Geometry check sheet. Reference: the model listing, model coordinates, mm. A direction names the side the tool comes from. Round coordinates to 2 decimals unless told otherwise and drop trailing zeros. Write each loop counter-clockwise with the first axis right and the second up, starting at its lowest first coordinate (ties: lowest second). Pieces come first, ordered by that corner, then holes.
from build123d import *

# Parameters (mm, degrees)
ESQUISSE1_R             = 2.25
BOSS_EXTRU_1_DEPTH      = 5
BOSS_EXTRU_2_START      = -21
BOSS_EXTRU_2_DEPTH      = 21
ESQUISSE4_W             = 13
ESQUISSE4_H             = 46
ENL_V_MAT_EXTRU_2_DEPTH = 16
ESQUISSE9_W             = 16
ESQUISSE9_H             = 36
BOSS_EXTRU_3_DEPTH      = 3
ESQUISSE10_W            = 4
ESQUISSE10_H            = 16
ENL_V_MAT_EXTRU_6_DEPTH = 43
CONG_1_R                = 2
ESQUISSE11_R            = 2.1
ENL_V_MAT_EXTRU_7_DEPTH = 43


with BuildPart() as part:
    # Esquisse1 → Boss.-Extru.1 (new body)
    with BuildSketch(Plane.XY):
        with BuildLine():
            Line((-7.4, 36), (-7.4, 0))
            Line((-7.4, 0), (7, 0))
            ThreePointArc((7, 0), (9.121320344, 0.878679656), (10, 3))
            Line((10, 3), (10, 33))
            ThreePointArc((10, 33), (9.121320344, 35.121320344), (7, 36))
            Line((7, 36), (-7.4, 36))
        make_face()
        with Locations((2, 8)):
            Circle(ESQUISSE1_R, mode=Mode.SUBTRACT)
        with Locations((2, 28)):
            Circle(ESQUISSE1_R, mode=Mode.SUBTRACT)
    extrude(amount=BOSS_EXTRU_1_DEPTH)

    # Esquisse2 → Boss.-Extru.2 (add)
    with BuildSketch(Plane.XY.offset(5).offset(BOSS_EXTRU_2_START)):
        with BuildLine():
            Line((10, 3), (10, 33))
            ThreePointArc((10, 33), (9.121320344, 35.121320344), (7, 36))
            Line((7, 36), (11, 36))
            Line((11, 36), (11, 41))
            Line((11, 41), (24, 41))
            Line((24, 41), (24, -5))
            Line((24, -5), (11, -5))
            Line((11, -5), (11, 0))
            Line((11, 0), (7, 0))
            ThreePointArc((7, 0), (9.121320344, 0.878679656), (10, 3))
        make_face()
    extrude(amount=BOSS_EXTRU_2_DEPTH)

    # Esquisse4 → Enlèv. mat.-Extru.2 (cut)
    with BuildSketch(Plane.XY.offset(5)):
        with Locations((17.5, 18)):
            Rectangle(ESQUISSE4_W, ESQUISSE4_H)
    extrude(amount=-ENL_V_MAT_EXTRU_2_DEPTH, mode=Mode.SUBTRACT)

    # Esquisse9 → Boss.-Extru.3 (add)
    with BuildSketch(Plane(origin=(11, 0, 0), x_dir=(0, 0, -1), z_dir=(1, 0, 0))):
        with Locations((3, 18)):
            Rectangle(ESQUISSE9_W, ESQUISSE9_H)
    extrude(amount=BOSS_EXTRU_3_DEPTH)

    # Esquisse10 → Enlèv. mat.-Extru.6 (cut)
    with BuildSketch(Plane(origin=(0, 36, 0), x_dir=(1, 0, 0), z_dir=(0, 1, 0))):
        with Locations((9, 8)):
            Rectangle(ESQUISSE10_W, ESQUISSE10_H)
    extrude(amount=-ENL_V_MAT_EXTRU_6_DEPTH, mode=Mode.SUBTRACT)

    # Congé1
    cong_1_edges = [part.edges().sort_by_distance(p)[0] for p in [
        (-7.4, 0, 2.5),
        (-7.4, 36, 2.5),
    ]]
    fillet(cong_1_edges, radius=CONG_1_R)

    # Esquisse11 → Enlèv. mat.-Extru.7 (cut)
    with BuildSketch(Plane.XY.offset(-11)):
        with Locations((19, 29)):
            Circle(ESQUISSE11_R)
        with Locations((19, 7)):
            Circle(ESQUISSE11_R)
    extrude(amount=-ENL_V_MAT_EXTRU_7_DEPTH, mode=Mode.SUBTRACT)


solid = part.part
1. Depth check by flat-ended pin: pin 1 Ø14.5 at (x, y) = (-0.5, 23.5) entering from -Z; pin 2 Ø4 at (x, y) = (2, 28) entering from -Z; pin 3 Ø8 at (y, z) = (26.5, -3.5) entering from +X; pin 4 Ø1 at (y, z) = (8, -8) entering from -X. Enter the tip coordinate at first touch or a pass-through.
2. Section check D-D (x = 13.5). Record the cut outline in (y, z), plus the area to 3 significant figures.
3. Section check B-B (z = 0.5). Record the cut outline in (x, y).
4. Access from +Z, -Z, +X, -X, +Y, -Y to the whole of each face (thin tool, end or side, straight path). Record for faces 1 (the face through (21.003, 7.631, -13.465)), 2 (the face through (6, 36, 1)), 3 (the face through (2, 18, 0)), 4 (the face through (14, 18, -3)).
5. Section check A-A (x = 19). Record the cut outline in (y, z), plus the area to 3 significant figures.
6. Section check C-C (y = 29). Record the cut outline in (x, z), plus the area to 3 significant figures.
7. Release check for a two-part mould opening along Y. For faces 5 (the face through (-6.83, 35.4, 2.54)), 6 (the face through (24, 18, -14)), 7 (the face through (1.512, 25.804, 2.465)), 8 (the face through (6, 0, 1)) record: +Y half, -Y half, draft (parallel to the pull), parting line (faces both ways), or undercut.
8. Scan lines: line 1 along Y through (x, z) = (19, -14); line 2 along Y through (x, z) = (2, 3.25); line 3 along X through (y, z) = (23, 0.25). Record each from-to range of solid material in increasing order.
Results below:
1. pin 1: stops at z = 0
1. pin 2: passes through
1. pin 3: stops at x = 14
1. pin 4: stops at x = 11
2. outline: (-5, -16) - (41, -16) - (41, -11) - (36, -11) - (36, 5) - (0, 5) - (0, -11) - (-5, -11) - close
2. area: 806 mm2
3. outline: (-7.4, 2) arc R2 ccw to (-5.4, 0) - (14, 0) - (14, 36) - (-5.4, 36) arc R2 ccw to (-7.4, 34) - close; hole circle Ø4.5 at (2, 8); hole circle Ø4.5 at (2, 28)
4. face 1: +Z, -Z
4. face 2: +Z, +X, -X, +Y
4. face 3: -Z, -X, +Y, -Y
4. face 4: +Z, +X, +Y, -Y
5. outline: (-5, -16) - (4.9, -16) - (4.9, -11) - (-5, -11) - close; (9.1, -16) - (26.9, -16) - (26.9, -11) - (9.1, -11) - close; (31.1, -16) - (41, -16) - (41, -11) - (31.1, -11) - close
5. area: 188 mm2
6. outline: (-7.4, 0) - (-0.02, 0) - (-0.02, 5) - (-7.4, 5) - close; (4.02, 0) - (11, 0) - (11, -16) - (16.9, -16) - (16.9, -11) - (14, -11) - (14, 5) - (4.02, 5) - close; (21.1, -16) - (24, -16) - (24, -11) - (21.1, -11) - close
6. area: 164 mm2
7. face 5: +Y half
7. face 6: draft
7. face 7: undercut
7. face 8: -Y half
8. line 1: y = -5 to 4.9, 9.1 to 26.9, 31.1 to 41
8. line 2: y = 0 to 5.75, 10.25 to 25.75, 30.25 to 36
8. line 3: x = -7.4 to 14
